The listing builds one solid part. Answer for the finished solid, in the listing's coordinates (mm). A direction names the side the tool comes from. Coordinates: 2 decimals unless noted, no trailing zeros. Order: outer loops, then holes, each group sorted by start corner. A loop starts at its lowest first (then second) coordinate and runs counter-clockwise, first axis right, second up.
from build123d import *

# Parameters (mm, degrees)
BOSS_EXTRUDE1_DEPTH = 3


with BuildPart() as part:
    # Sketch1 → Boss-Extrude1 (new body)
    with BuildSketch(Plane(origin=(0, 0, 0), x_dir=(1, 0, 0), z_dir=(0, 1, 0))):
        with BuildLine():
            Line((0, 0), (0, 10.5))
            ThreePointArc((0, 10.5), (0.732233047, 12.267766953), (2.5, 13))
            Line((2.5, 13), (12.5, 13))
            ThreePointArc((12.5, 13), (14.267766953, 12.267766953), (15, 10.5))
            Line((15, 10.5), (15, 0))
            Line((15, 0), (10, 0))
            Line((10, 0), (10, 3))
            Line((10, 3), (5, 3))
            Line((5, 3), (5, 0))
            Line((5, 0), (0, 0))
        make_face()
        Polygon((5.767949192, 5), (9.232050808, 5), (10.964101615, 8), (9.232050808, 11), (5.767949192, 11), (4.035898385, 8), align=None, mode=Mode.SUBTRACT)
    extrude(amount=BOSS_EXTRUDE1_DEPTH)


solid = part.part
1) Section C-C (z = -9) is taken. Give the vertices of the cut face in (x, y), then the cut area to 3 significant figures.
2) A tool of negligible diameter and unlimited length cuts with its end or side. For faces 1 (the face through (8, 1, -3)), 2 (the face through (7, 1, -5)), 3 (the face through (8, 3, -4)), from which of +Z, -Z, +X, -X, +Y, -Y can it reach the whole face along a straight path? Write none if from no direction.
3) Section B-B (y = 2.4) is taken. Give the vertices of the cut face in (x, z).
4) Section D-D (z = -11.75) is taken. Give the vertices of the cut face in (x, y).
5) Each of these flat-tipped pins is pushed along its axis until it touches: P1, Ø1.5, axis at x = 8, y = 1.5, coming from the +Z side; P2, Ø4, axis at x = 11, z = -10, coming from the -Y side. Where does it stop, or does it pass through?
6) Section A-A (x = 9) is taken. Give the vertices of the cut face in (y, z), then the cut area to 3 significant figures.
7) Consider L1, parallel to X at y = 0.3, z = -2.5; L2, parallel to Z at x = 6, y = 1.6; L3, parallel to X at y = 0.65, z = -7.5. Determine where each line is inside the solid, lowest interval first.
8) Determine the mould class of faces 4 (the face through (10.1, 1.5, -6.5)), 5 (the face through (10, 1, -1)), 6 (the face through (13, 1, 0)) for opening direction Z: released by +Z, released by -Z, zero draft, split by the parting line, or undercut.
Filled sheet:
1. outline: (0, 0) - (4.61, 0) - (4.61, 3) - (0, 3) - close; (10.39, 0) - (15, 0) - (15, 3) - (10.39, 3) - close
1. area: 27.7 mm2
2. face 1: +Z, +Y, -Y
2. face 2: +Y, -Y
2. face 3: +Z, -Z, +X, -X, +Y
3. outline: (0, -10.5) arc R2.5 ccw to (2.5, -13) - (12.5, -13) arc R2.5 ccw to (15, -10.5) - (15, 0) - (10, 0) - (10, -3) - (5, -3) - (5, 0) - (0, 0) - close; hole (4.04, -8) - (5.77, -11) - (9.23, -11) - (10.96, -8) - (9.23, -5) - (5.77, -5) - close
4. outline: (0.33, 0) - (14.67, 0) - (14.67, 3) - (0.33, 3) - close
5. P1: stops at z = -3
5. P2: stops at y = 0
6. outline: (0, -13) - (3, -13) - (3, -11) - (0, -11) - close; (0, -5) - (3, -5) - (3, -3) - (0, -3) - close
6. area: 12.0 mm2
7. L1: x = 0 to 5, 10 to 15
7. L2: z = -13 to -11, -5 to -3
7. L3: x = 0 to 4.32, 10.68 to 15
8. face 4: undercut
8. face 5: zero draft
8. face 6: released by +Z
